Answer from the drawing. Dimensions are ordinates in mm from the lowest x, y and z of the part. A direction names the side the tool comes from. Give positions to 0.01 mm unless a question says otherwise; leave off trailing zeros. Write each loop counter-clockwise with the first axis right and the second up, starting at its lowest first coordinate (ties: lowest second). Pieces come first, ordered by that corner, then holes. Notation, with made-up numbers: (-30, 21) -> (-2, 21) arc R16 ccw to (-2, 39) -> close; hole circle Ø3 at (13, 86.25). An arc over 180 degrees is marked (long way). Put each result on its own line as item: value. Start each with the question number.
1) Find the intervals of material crossed by line 1 along Y through (x, z) = (8.75, 1); line 2 along X through (y, z) = (7, 3); line 3 along Z through (x, y) = (7.25, 12), in increasing order. Write a range as from..to.
2) For the marked faces 5 and 6, determine the directions among +Z, -Z, +X, -X, +Y, -Y from which every point of the face is accessible in a straight line to the end or side of a thin tool.
3) Flat-ended cylindrical pins translate along their axes: pin 1 Ø1 at (x, y) = (12.5, 6.5) entering from +Z; pin 2 Ø4 at (x, y) = (17, 5.5) entering from -Z; pin 3 Ø1 at (y, z) = (8, 12) entering from -X. Find the tip coordinate at first contact, or state that the pin passes through.
4) A cutting plane is placed at D-D (x = 27.5). Write down the section's boundary in (y, z), then the cut area to 3 significant figures.
5) A cutting plane is placed at C-C (z = 13.25). Write down the section's boundary in (x, y) (3 decimals).
6) A cutting plane is placed at A-A (x = 8.89). Write down the section's boundary in (y, z) (3 decimals).
7) A cutting plane is placed at B-B (y = 3.5). Write down the section's boundary in (x, z).
8) For a pull along Y with two mould halves and no side action, classify the marked faces 1, 2, 3 and 4 as released by +Y, released by -Y, zero draft, split by the parting line, or undercut.
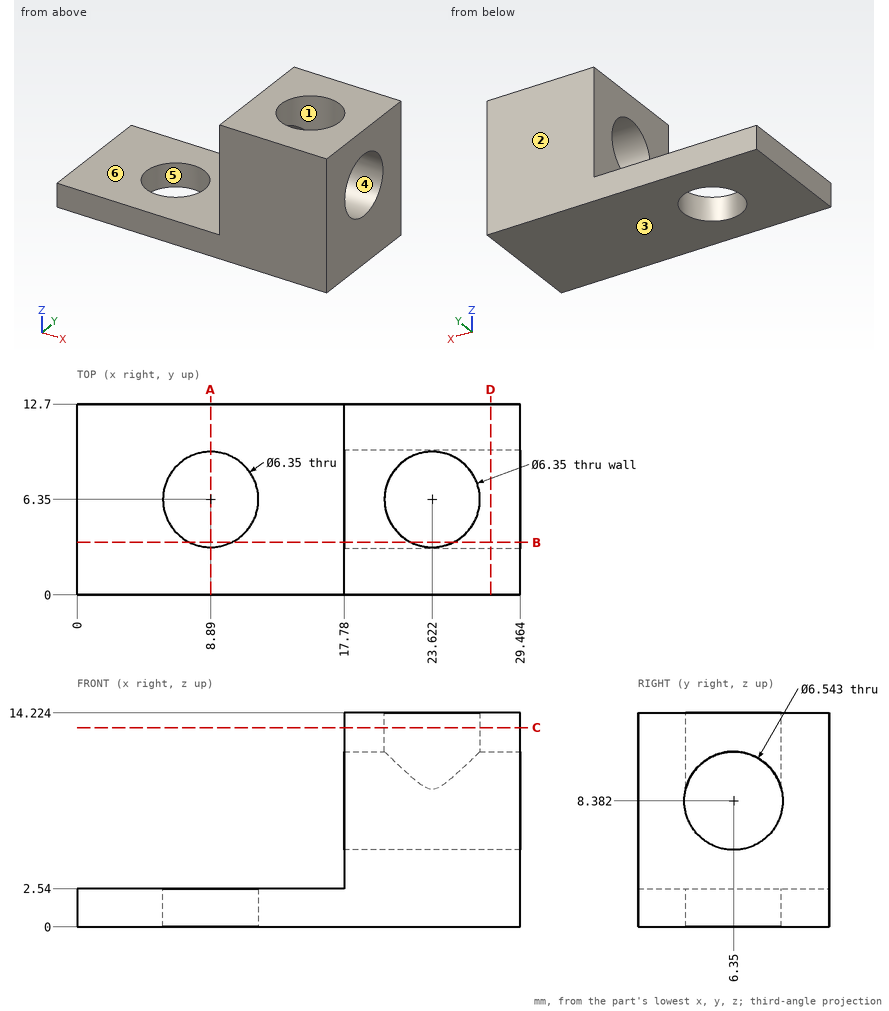
Reply:
1. line 1: y = 0..3.18, 9.52..12.7
1. line 2: x = 17.78..29.46
1. line 3: z = 0..2.54
2. face 5: +Z, -Z
2. face 6: +Z, -X, +Y, -Y
3. pin 1: stops at z = 2.54
3. pin 2: stops at z = 0
3. pin 3: stops at x = 17.78
4. outline: (0, 0) -> (12.7, 0) -> (12.7, 14.22) -> (0, 14.22) -> close; hole circle Ø6.54 at (6.35, 8.38)
4. area: 147 mm2
5. outline: (17.78, 0) -> (29.464, 0) -> (29.464, 12.7) -> (17.78, 12.7) -> close; hole circle Ø6.35 at (23.622, 6.35)
6. outline: (0, 0) -> (3.175, 0) -> (3.175, 2.54) -> (0, 2.54) -> close; (9.525, 0) -> (12.7, 0) -> (12.7, 2.54) -> (9.525, 2.54) -> close
7. outline: (0, 0) -> (7.49, 0) -> (7.49, 2.54) -> (0, 2.54) -> close; (10.29, 0) -> (29.46, 0) -> (29.46, 6.78) -> (17.78, 6.78) -> (17.78, 2.54) -> (10.29, 2.54) -> close; (17.78, 9.99) -> (22.22, 9.99) -> (22.22, 14.22) -> (17.78, 14.22) -> close; (25.02, 9.99) -> (29.46, 9.99) -> (29.46, 14.22) -> (25.02, 14.22) -> close
8. face 1: undercut
8. face 2: released by +Y
8. face 3: zero draft
8. face 4: undercut
